Verification items for the finished model (mm, model axes). A direction names the side the tool comes from. Coordinates: 2 decimals unless noted, no trailing zeros. Write each loop counter-clockwise with the first axis right and the second up, starting at its lowest first coordinate (ties: lowest second). Pieces come first, ordered by that corner, then holes. Notation, with made-up numbers: (-31.5, -5.5) -> (15.5, -5.5) arc R22 ccw to (15.5, 15.5) -> close; hole circle Ø8 at (-21, 31.25). An arc over 180 degrees is marked (long way). Answer in a Markdown table with one row per item.
```python
from build123d import *

# Parameters (mm, degrees)
SALIENTE_EXTRUIR1_DEPTH  = 24
REDONDEO1_R              = 2
CROQUIS2_R               = 4.5
SALIENTE_EXTRUIR2_DEPTH  = 3.2
REDONDEO2_R              = 0.5
CROQUIS3_R               = 0.65
SALIENTE_EXTRUIR3_DEPTH  = 1
REDONDEO3_R              = 10
REDONDEO3_OF_SIMETR_A1_R = 10


with BuildPart() as part:
    # Croquis1 → Saliente-Extruir1 (new body)
    with BuildSketch(Plane.XY):
        with BuildLine():
            Line((7.09, 7.75), (-7.09, 7.75))
            ThreePointArc((-7.09, 7.75), (-10.25, 0), (-7.09, -7.75))
            Line((-7.09, -7.75), (7.09, -7.75))
            ThreePointArc((7.09, -7.75), (10.25, 0), (7.09, 7.75))
        make_face()
    extrude(amount=SALIENTE_EXTRUIR1_DEPTH)

    # Redondeo1
    redondeo1_edges = [part.edges().sort_by_distance(p)[0] for p in [
        (10.25, 0, 24),
        (0, 7.75, 24),
        (-10.25, 0, 24),
        (0, -7.75, 24),
    ]]
    fillet(redondeo1_edges, radius=REDONDEO1_R)

    # Croquis2 → Saliente-Extruir2 (add)
    with BuildSketch(Plane.XY.offset(24)):
        Circle(CROQUIS2_R)
    extrude(amount=SALIENTE_EXTRUIR2_DEPTH)

    # Redondeo2
    redondeo2_edges = [part.edges().sort_by_distance(p)[0] for p in [
        (-4.5, 0, 27.2),
    ]]
    fillet(redondeo2_edges, radius=REDONDEO2_R)

    # Croquis3 → Saliente-Extruir3 (add)
    with BuildSketch(Plane.XZ.offset(7.75)):
        with BuildLine():
            Line((-6.59, 22), (-11.59, 22))
            ThreePointArc((-11.59, 22), (-12.297106781, 21.707106781), (-12.59, 21))
            Line((-12.59, 21), (-12.59, 19.5))
            ThreePointArc((-12.59, 19.5), (-12.297106781, 18.792893219), (-11.59, 18.5))
            Line((-11.59, 18.5), (-6.59, 18.5))
            Line((-6.59, 18.5), (-6.59, 22))
        make_face()
        with Locations(Location((-11.09, 20.25, 0), (0, 0, 270))):
            Circle(CROQUIS3_R, mode=Mode.SUBTRACT)
    saliente_extruir3 = extrude(amount=SALIENTE_EXTRUIR3_DEPTH)

    # Redondeo3
    # the kernel refuses this fillet: 10 mm, written as the material it adds along each edge
    with BuildSketch(Plane(origin=(-6.59, -7.75, 18.5), x_dir=(1, 0, 0), z_dir=(0, 0, 1))) as redondeo3_piece_1:
        with BuildLine():
            CenterArc((4.358898944, -10), REDONDEO3_R, 90, 25.841932763)
            Line((0, -1), (-0.087177979, -0.82))
            ThreePointArc((-0.087177979, -0.82), (-0.2, -0.5), (-0.2, 0))
            Line((-0.2, 0), (0, 0.2))
            Line((0, 0.2), (4.358898944, 0.2))
            Line((4.358898944, 0.2), (4.358898944, 0))
        make_face()
    extrude(amount=3.5)

    # Simetría1: Saliente-Extruir3 across plane
    add(saliente_extruir3.mirror(Plane(origin=(0, 0, 0), x_dir=(0, 0, 1), z_dir=(1, 0, 0))))

    # Redondeo3 of Simetría1
    # the kernel refuses this fillet: 10 mm, written as the material it adds along each edge
    with BuildSketch(Plane(origin=(6.59, -7.75, 18.5), x_dir=(-1, 0, 0), z_dir=(0, 0, 1))) as redondeo3_of_simetr_a1_piece_1:
        with BuildLine():
            CenterArc((4.358898944, 10), REDONDEO3_OF_SIMETR_A1_R, 244.158067237, 25.841932763)
            Line((0, 1), (-0.087177979, 0.82))
            ThreePointArc((-0.087177979, 0.82), (-0.2, 0.5), (-0.2, 0))
            Line((-0.2, 0), (0, -0.2))
            Line((0, -0.2), (4.358898944, -0.2))
            Line((4.358898944, -0.2), (4.358898944, 0))
        make_face()
    extrude(amount=3.5)


solid = part.part
```
1. Section check A-A, the plane x = 11.09. Record the boundary of the cut face in (y, z), plus the area to 3 significant figures.
Geometry says:
| item | result |
|---|---|
| outline | (-8.75, 18.5) -> (-7.75, 18.5) -> (-7.75, 19.6) -> (-8.75, 19.6) -> close; (-8.75, 20.9) -> (-7.75, 20.9) -> (-7.75, 22) -> (-8.75, 22) -> close |
| area | 2.20 mm^2 |
2. Tool access check on faces 1 (the flat face through (-12.59, -8, 20)), 2 (the flat face through (-4, 3, 24)), 3 (the cylindrical face through (-4.436, -7.996, 20.226)), 4 (the flat face through (0, 7.75, 11)), 5 (the flat face through (-8, -8, 22)). Record the directions out of +Z, -Z, +X, -X, +Y, -Y that give a thin tool (end or side, any length) a straight path to the whole face; none if there is none.
Geometry says:
| item | result |
|---|---|
| face 1 | +Z, -Z, -X, +Y, -Y |
| face 2 | +Z |
| face 3 | +Z, -Z, -Y |
| face 4 | +Z, -Z, +X, -X, +Y |
| face 5 | +Z, +X, -X, -Y |
3. Section check D-D, the plane x = 0. Record the boundary of the cut face in (y, z), plus the area to 3 significant figures.
Geometry says:
| item | result |
|---|---|
| outline | (-7.75, 0) -> (7.75, 0) -> (7.75, 22) arc R2 ccw to (5.75, 24) -> (4.5, 24) -> (4.5, 26.7) arc R0.5 ccw to (4, 27.2) -> (-4, 27.2) arc R0.5 ccw to (-4.5, 26.7) -> (-4.5, 24) -> (-5.75, 24) arc R2 ccw to (-7.75, 22) -> close |
| area | 399 mm^2 |
4. Thickness scan on line 1 (X direction, y = -8.45, z = 20.25); line 2 (Z direction, x = 11.09, y = -8); line 3 (Z direction, x = -5.5, y = -5.25). Record the ranges inside material, lowest first. Write a range as from..to.
Geometry says:
| item | result |
|---|---|
| line 1 | -12.59..-11.74, -10.44..-5.91, 5.91..10.44, 11.74..12.59 |
| line 2 | 18.5..19.6, 20.9..22 |
| line 3 | 0..24 |
5. Depth check by flat-ended pin: P1, Ø1.2, axis at x = 11.09, z = 20.25, coming from the -Y side; P2, Ø1.1, axis at x = -8, y = -8, coming from the +Z side; P3, Ø1.1, axis at x = -6.5, y = -8.5, coming from the -Z side; P4, Ø8, axis at y = 4, z = 4, coming from the -X side. Enter the tip coordinate at first touch or a pass-through.
Geometry says:
| item | result |
|---|---|
| P1 | through |
| P2 | z = 22 |
| P3 | z = 18.5 |
| P4 | x = -10.25 |
6. Section check B-B, the plane z = 20.25. Record the boundary of the cut face in (x, y).
Geometry says:
| item | result |
|---|---|
| outline | (-12.59, -8.75) -> (-11.74, -8.75) -> (-11.74, -7.75) -> (-12.59, -7.75) -> close; (-10.44, -8.75) -> (-6.59, -8.75) arc R10 cw to (-2.23, -7.75) -> (2.23, -7.75) arc R10 cw to (6.59, -8.75) -> (10.44, -8.75) -> (10.44, -7.75) -> (7.09, -7.75) arc R11.08 ccw to (7.09, 7.75) -> (-7.09, 7.75) arc R11.08 ccw to (-7.09, -7.75) -> (-10.44, -7.75) -> close; (11.74, -8.75) -> (12.59, -8.75) -> (12.59, -7.75) -> (11.74, -7.75) -> close |
7. Section check C-C, the plane y = 0. Record the boundary of the cut face in (x, z).
Geometry says:
| item | result |
|---|---|
| outline | (-10.25, 0) -> (10.25, 0) -> (10.25, 22) arc R2 ccw to (8.25, 24) -> (4.5, 24) -> (4.5, 26.7) arc R0.5 ccw to (4, 27.2) -> (-4, 27.2) arc R0.5 ccw to (-4.5, 26.7) -> (-4.5, 24) -> (-8.25, 24) arc R2 ccw to (-10.25, 22) -> close |
8. Mould release check, pull along Y, two halves, no side actions. Record for faces 6 (the flat face through (10, -7.75, 20)), 7 (the cylindrical face through (4.5, -8.01, 20.23)), 8 (the cylindrical face through (-12.305, -8.243, 18.801)): released by +Y, released by -Y, zero draft, split by the parting line, or undercut.
Geometry says:
| item | result |
|---|---|
| face 6 | undercut |
| face 7 | released by -Y |
| face 8 | zero draft |
